Verification items for the finished model (mm, model axes). Face numbers are marked on the shaded views. A direction names the side the tool comes from. Coordinates: 2 decimals unless noted, no trailing zeros. Write each loop counter-clockwise with the first axis right and the second up, starting at its lowest first coordinate (ties: lowest second). Pieces come first, ordered by that corner, then holes. Notation, with made-up numbers: (38, 88) -> (42, 88) arc R25 ccw to (42, 111) -> close; hole circle Ø6 at (19.25, 41). An arc over 180 degrees is marked (long way). Answer in a Markdown table with one row per item.
Autodesk Inventor part; units mm, degrees
ref_plane "YZ Plane" through (0, 0, 0) normal (1, 0, 0) x (0, 1, 0)
ref_plane "XZ Plane" through (0, 0, 0) normal (0, 1, 0) x (-1, 0, 0)
ref_plane "XY Plane" through (0, 0, 0) normal (0, 0, 1) x (1, 0, 0)
sketch "Skizze1" plane through (0, 0, 0) normal (0, 1, 0) x (-1, 0, 0)
  line L0 (0, 0) -> (-109.21, 0)
  line L1 (-109.21, 0) -> (-109.21, 96.9)
  line L2 (-109.21, 96.9) -> (0, 96.9)
  line L3 (0, 96.9) -> (0, 0)
  dimension "d5" = 109.21
  dimension "d6" = 96.9
extrude "Extrusion1" add sketch "Skizze1" along normal blind 12
sketch "Skizze2" plane through (0, 12, 0) normal (0, 1, 0) x (1, 0, 0)
  line L0 (7.6, 0) -> (102.6, 0)
  line L1 (102.6, 0) -> (102.6, -56.9)
  line L2 (96.6, -62.9) -> (13.6, -62.9)
  line L3 (7.6, -56.9) -> (7.6, 0)
  arc A0 (7.6, -56.9) -> (13.6, -62.9) centre (13.6, -56.9) ccw
  arc A1 (96.6, -62.9) -> (102.6, -56.9) centre (96.6, -56.9) ccw
  line L4 (0, 0) -> (0, -96.9)
  line L5 (109.21, 0) -> (0, 0)
  dimension "d2" = 6
  dimension "d7" = 7.6
  dimension "d8" = 62.9
  dimension "d9" = 95
extrude "Extrusion2" cut sketch "Skizze2" against normal through all
sketch "Skizze3" plane through (0, 12, 0) normal (0, 1, 0) x (1, 0, 0)
  line L0 (7.6, -56.9) -> (7.6, 0)
  line L1 (7.6, 0) -> (0, 0)
  line L2 (0, 0) -> (0, -96.9)
  line L3 (0, -96.9) -> (109.21, -96.9)
  line L4 (109.21, -96.9) -> (109.21, 0)
  line L5 (109.21, 0) -> (102.6, 0)
  line L6 (102.6, 0) -> (102.6, -56.9)
  arc A0 (96.6, -62.9) -> (102.6, -56.9) centre (96.6, -56.9) ccw
  line L7 (96.6, -62.9) -> (13.6, -62.9)
  arc A1 (7.6, -56.9) -> (13.6, -62.9) centre (13.6, -56.9) ccw
  line L8 (102.6, 0) -> (102.7, 0)
  line L9 (102.7, 0) -> (102.7, -35)
  line L10 (102.7, -35) -> (102.6, -35)
  line L11 (102.6, -35) -> (102.6, 0)
  line L12 (7.6, 0) -> (7.6, -56.9)
  line L13 (7.6, 0) -> (7.5, 0)
  line L14 (7.5, 0) -> (7.5, -40)
  line L15 (7.5, -40) -> (7.6, -40)
  line L16 (7.6, -40) -> (7.6, 0)
  point P0 (102.6, -35)
  dimension "d10" = 0.1
  dimension "d11" = 35
  dimension "d12" = 0.1
extrude "Extrusion3" cut sketch "Skizze3" against normal through all contours L15 L14 L1 L0 | L6 L5 L9 L10
properties part number "30_XYTable_Aliexpress_CAM_cutout"
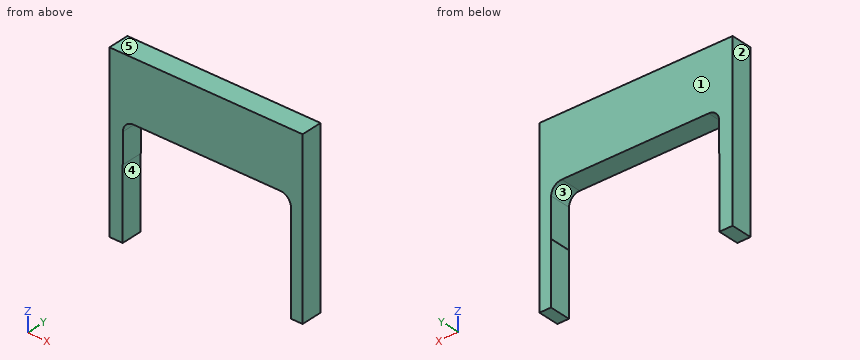
1. Tool access check on the marked faces 4 and 5. Record the directions out of +Z, -Z, +X, -X, +Y, -Y that give a thin tool (end or side, any length) a straight path to the whole face; none if there is none.
Geometry says:
| item | result |
|---|---|
| face 4 | -Z, +Y, -Y |
| face 5 | +Z, +X, -X, +Y, -Y |
2. Thickness scan on line 1 (X direction, y = 6, z = 22.5); line 2 (X direction, y = 3.5, z = 38); line 3 (Z direction, x = 67.5, y = 10.5). Record the ranges inside material, lowest first. Write a range as from..to.
Geometry says:
| item | result |
|---|---|
| line 1 | 0..7.5, 102.7..109.21 |
| line 2 | 0..7.5, 102.6..109.21 |
| line 3 | 62.9..96.9 |
3. Mould release check, pull along X, two halves, no side actions. Record for the marked faces 1, 2 and 3: released by +X, released by -X, zero draft, split by the parting line, or undercut.
Geometry says:
| item | result |
|---|---|
| face 1 | zero draft |
| face 2 | released by -X |
| face 3 | undercut |
4. Section check B-B, the plane y = 9.5. Record the boundary of the cut face in (x, z), plus the area to 3 significant figures.
Geometry says:
| item | result |
|---|---|
| outline | (0, 0) -> (7.5, 0) -> (7.5, 40) -> (7.6, 40) -> (7.6, 56.9) arc R6 cw to (13.6, 62.9) -> (96.6, 62.9) arc R6 cw to (102.6, 56.9) -> (102.6, 35) -> (102.7, 35) -> (102.7, 0) -> (109.21, 0) -> (109.21, 96.9) -> (0, 96.9) -> close |
| area | 4,610 mm^2 |
5. Section check D-D, the plane x = 43.5. Record the boundary of the cut face in (y, z).
Geometry says:
| item | result |
|---|---|
| outline | (0, 62.9) -> (12, 62.9) -> (12, 96.9) -> (0, 96.9) -> close |
6. Section check C-C, the plane z = 31.5. Record the boundary of the cut face in (x, y), plus the area to 3 significant figures.
Geometry says:
| item | result |
|---|---|
| outline | (0, 0) -> (7.5, 0) -> (7.5, 12) -> (0, 12) -> close; (102.7, 0) -> (109.21, 0) -> (109.21, 12) -> (102.7, 12) -> close |
| area | 168 mm^2 |
7. Section check A-A, the plane z = 42.5. Record the boundary of the cut face in (x, y).
Geometry says:
| item | result |
|---|---|
| outline | (0, 0) -> (7.6, 0) -> (7.6, 12) -> (0, 12) -> close; (102.6, 0) -> (109.21, 0) -> (109.21, 12) -> (102.6, 12) -> close |
8. Depth check by flat-ended pin: P1, Ø3.5, axis at x = 75.5, y = 5, coming from the -Z side; P2, Ø6, axis at y = 7.5, z = 44.5, coming from the -X side; P3, Ø10, axis at x = 24.5, z = 56.5, coming from the -Y side. Enter the tip coordinate at first touch or a pass-through.
Geometry says:
| item | result |
|---|---|
| P1 | z = 62.9 |
| P2 | x = 0 |
| P3 | through |
